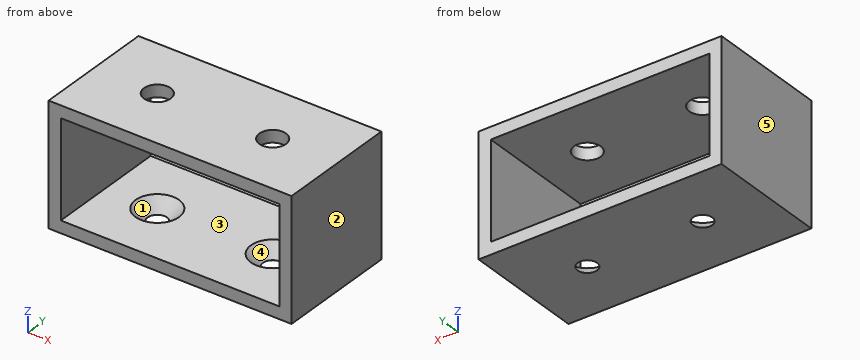
from build123d import *

# Parameters (mm, degrees)
SKETCH_W          = 50
SKETCH_H          = 25
PAD_DEPTH         = 25
SKETCH001_W       = 45
SKETCH001_H       = 20
POCKET_DEPTH      = 0.001
POCKET_DEPTH_BACK = 25.001
SKETCH002_R       = 2.75
POCKET001_DEPTH   = 3.5
SKETCH003_R       = 2
POCKET002_DEPTH   = 2.5
CHAMFER_SIZE      = 2.485


with BuildPart() as part:
    # Sketch → Pad (new body)
    with BuildSketch(Plane.XZ):
        Rectangle(SKETCH_W, SKETCH_H)
    extrude(amount=PAD_DEPTH)

    # Sketch001 → Pocket (cut, two sides)
    with BuildSketch(Plane.XZ) as pocket_sk:
        Rectangle(SKETCH001_W, SKETCH001_H)
    extrude(amount=-POCKET_DEPTH, mode=Mode.SUBTRACT)
    extrude(pocket_sk.sketch, amount=POCKET_DEPTH_BACK, mode=Mode.SUBTRACT)

    # Sketch002 (on DatumPlane) → Pocket001 (cut)
    with BuildSketch(Plane(origin=(0, 0, 12.5), x_dir=(-1, 0, 0), z_dir=(0, 0, 1))):
        with Locations((-11.875, 12.5)):
            Circle(SKETCH002_R)
        with Locations((11.875, 12.5)):
            Circle(SKETCH002_R)
    extrude(amount=-POCKET001_DEPTH, mode=Mode.SUBTRACT)

    # Sketch003 (on DatumPlane) → Pocket002 (cut)
    with BuildSketch(Plane(origin=(0, 0, -10), x_dir=(-1, 0, 0), z_dir=(0, 0, 1))):
        with Locations((-11.875, 12.5)):
            Circle(SKETCH003_R)
        with Locations((11.875, 12.5)):
            Circle(SKETCH003_R)
    extrude(amount=-POCKET002_DEPTH, mode=Mode.SUBTRACT)

    # Chamfer
    chamfer_edges = [part.edges().sort_by_distance(p)[0] for p in [
        (-9.875, -12.5, -10),
        (13.875, -12.5, -10),
    ]]
    chamfer(chamfer_edges, length=CHAMFER_SIZE)


solid = part.part
Model file for the job. Use its own axes, mm. Face numbers are marked on the shaded views. A direction names the side the tool comes from. Round coordinates to 2 decimals unless told otherwise and drop trailing zeros. Loops run counter-clockwise (first coordinate to the right, second up) from the corner with the lowest first, then second, coordinate; pieces in that order, holes last.
1. Band-saw the part on C-C, the plane z = 8.5. List the corners of the cut face in (x, y).
Check values:
outline: (-25, -25) - (-22.5, -25) - (-22.5, 0) - (-25, 0) - close; (22.5, -25) - (25, -25) - (25, 0) - (22.5, 0) - close
2. Band-saw the part on B-B, the plane y = -19.25. List the corners of the cut face in (x, z), and give its area (3 significant figures).
Check values:
outline: (-25, -12.5) - (25, -12.5) - (25, 12.5) - (-25, 12.5) - close; hole (-22.5, -10) - (22.5, -10) - (22.5, 10) - (-22.5, 10) - close
area: 350 mm2
3. Mould opens along Y. For the marked faces 1 and 2 say: +Y half, -Y half, draft (parallel to the pull), parting line (faces both ways), or undercut.
Check values:
face 1: undercut
face 2: draft
4. Wall check: probe 1 along X at (y, z) = (-12.5, 11.2) (3 decimals); probe 2 along Z at (x, y) = (3, -15.25); probe 3 along X at (y, z) = (-20, 5.25). Give the ranges that are in metal, low to high.
Check values:
probe 1: x = -25 to -14.625, -9.125 to 9.125, 14.625 to 25
probe 2: z = -12.5 to -10, 10 to 12.5
probe 3: x = -25 to -22.5, 22.5 to 25
5. Band-saw the part on A-A, the plane x = 3.5. List the corners of the cut face in (y, z).
Check values:
outline: (-25, -12.5) - (0, -12.5) - (0, -10) - (-25, -10) - close; (-25, 10) - (0, 10) - (0, 12.5) - (-25, 12.5) - close
6. Tool access for the marked faces 3, 4 and 5: list every direction of +Z, -Z, +X, -X, +Y, -Y with a clear straight run to the whole face (end or side of a thin tool).
Check values:
face 3: +Y, -Y
face 4: none
face 5: +Z, -Z, -X, +Y, -Y
7. Band-saw the part on D-D, the plane y = -12.5. List the corners of the cut face in (x, z) (3 decimals), and give its area (3 significant figures).
Check values:
outline: (-25, -12.5) - (-13.875, -12.5) - (-13.875, -12.485) - (-16.36, -10) - (-22.5, -10) - (-22.5, 10) - (-14.625, 10) - (-14.625, 12.5) - (-25, 12.5) - close; (-9.875, -12.5) - (9.875, -12.5) - (9.875, -12.485) - (7.39, -10) - (-7.39, -10) - (-9.875, -12.485) - close; (-9.125, 10) - (9.125, 10) - (9.125, 12.5) - (-9.125, 12.5) - close; (13.875, -12.5) - (25, -12.5) - (25, 12.5) - (14.625, 12.5) - (14.625, 10) - (22.5, 10) - (22.5, -10) - (16.36, -10) - (13.875, -12.485) - close
area: 290 mm2
8. Drop a flat-ended pin along its axis: P1, Ø5, axis at x = -11.875, y = -12.5, coming from the +Z side (3 decimals). Give the stop position or say it passes through.
Check values:
P1: stops at z = -11.985
